Can you work these out from the drawing? Everything is in mm from the part's minimum corner. A direction names the side the tool comes from. Round coordinates to 2 decimals unless told otherwise and drop trailing zeros. Loops run counter-clockwise (first coordinate to the right, second up) from the corner with the lowest first, then second, coordinate; pieces in that order, holes last. Notation, with made-up numbers: (16.5, 73) -> (72.5, 73) arc R10 ccw to (72.5, 88) -> close; hole circle Ø8 at (32.25, -29.75). An arc over 180 degrees is marked (long way). One line per item, written item: value.
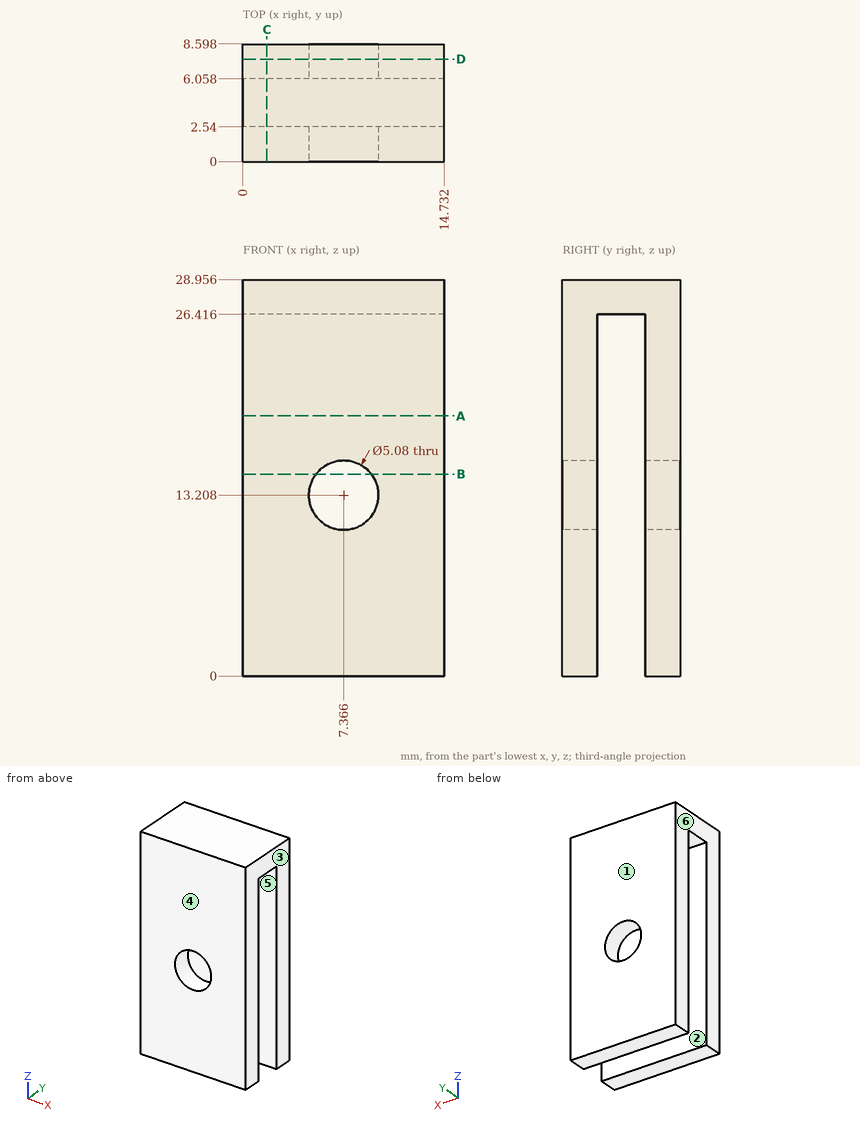
(1) If we section it at B-B, the plane z = 14.75: Please give me the cut outline in (x, y).
Recorded:
outline: (0, 0) -> (5.35, 0) -> (5.35, 2.54) -> (0, 2.54) -> close; (0, 6.06) -> (5.35, 6.06) -> (5.35, 8.6) -> (0, 8.6) -> close; (9.38, 0) -> (14.73, 0) -> (14.73, 2.54) -> (9.38, 2.54) -> close; (9.38, 6.06) -> (14.73, 6.06) -> (14.73, 8.6) -> (9.38, 8.6) -> close
(2) Thinking about a two-plate mould opening in Y: for the marked faces 1, 2, 3 and 4, which applies, released by +Y, released by -Y, zero draft, split by the parting line, or undercut?
Recorded:
face 1: released by +Y
face 2: undercut
face 3: zero draft
face 4: released by -Y
(3) If we section it at C-C, the plane x = 1.75: Please give me the cut outline in (y, z).
Recorded:
outline: (0, 0) -> (2.54, 0) -> (2.54, 26.42) -> (6.06, 26.42) -> (6.06, 0) -> (8.6, 0) -> (8.6, 28.96) -> (0, 28.96) -> close
(4) If I drill on L1, parallel to Y at x = 3, z = 19; L2, parallel to X at y = 0.75, z = 14.5; L3, parallel to Z at x = 3, y = 4.5, over which ranges is the centre line in solid material (lowest first)?
Recorded:
L1: 0 to 2.54, 6.06 to 8.6
L2: 0 to 5.18, 9.55 to 14.73
L3: 26.42 to 28.96
(5) If we section it at D-D, the plane y = 7.5: Please give me the cut outline in (x, z).
Recorded:
outline: (0, 0) -> (14.73, 0) -> (14.73, 28.96) -> (0, 28.96) -> close; hole circle Ø5.08 at (7.37, 13.21)
(6) If we section it at A-A, the plane z = 19: Please give me the cut outline in (x, y).
Recorded:
outline: (0, 0) -> (14.73, 0) -> (14.73, 2.54) -> (0, 2.54) -> close; (0, 6.06) -> (14.73, 6.06) -> (14.73, 8.6) -> (0, 8.6) -> close
(7) For the marked faces 5 and 6, which set-ups out of +Z, -Z, +X, -X, +Y, -Y let a thin tool reach every point of the face, with its end or its side?
Recorded:
face 5: -Z, +X, -X
face 6: +Z, -Z, -X, +Y, -Y
